```python
from build123d import *

# Parameters (mm, degrees)
ESBO_O1_W                = 180
ESBO_O1_H                = 80
RESSALTO_EXTRUS_O1_DEPTH = 2
ESBO_O2_R                = 1.5
CORTE_EXTRUS_O1_DEPTH    = 2
ESBO_O3_W                = 22
ESBO_O3_H                = 2.5
CORTE_EXTRUS_O2_DEPTH    = 2
FILETE4_R                = 1.25
FILETE5_R                = 1.25
FILETE6_R                = 1.25
FILETE7_R                = 1.25


with BuildPart() as part:
    # Esboço1 → Ressalto-extrusão1 (new body)
    with BuildSketch(Plane.XY):
        with Locations((90, -40)):
            Rectangle(ESBO_O1_W, ESBO_O1_H)
    extrude(amount=RESSALTO_EXTRUS_O1_DEPTH)

    # Esboço2 → Corte-extrusão1 (cut)
    with BuildSketch(Plane.XY.offset(2)):
        with Locations((5.5, -58.5)):
            Circle(ESBO_O2_R)
        with Locations((5.5, -21.5)):
            Circle(ESBO_O2_R)
        with Locations((174.5, -21.5)):
            Circle(ESBO_O2_R)
        with Locations((174.5, -58.5)):
            Circle(ESBO_O2_R)
    extrude(amount=-CORTE_EXTRUS_O1_DEPTH, mode=Mode.SUBTRACT)

    # Esboço3 → Corte-extrusão2 (cut)
    with BuildSketch(Plane.XY):
        with Locations((90, -12.25)):
            Rectangle(ESBO_O3_W, ESBO_O3_H)
        with Locations((90, -67.75)):
            Rectangle(ESBO_O3_W, ESBO_O3_H)
    extrude(amount=CORTE_EXTRUS_O2_DEPTH, mode=Mode.SUBTRACT)

    # Filete4
    filete4_edges = [part.edges().sort_by_distance(p)[0] for p in [
        (79, -11, 1),
        (79, -13.5, 1),
    ]]
    fillet(filete4_edges, radius=FILETE4_R - 0.0001)  # a hair under: the kernel refuses the full size

    # Filete5
    filete5_edges = [part.edges().sort_by_distance(p)[0] for p in [
        (101, -13.5, 1),
        (101, -11, 1),
    ]]
    fillet(filete5_edges, radius=FILETE5_R - 0.0001)  # a hair under: the kernel refuses the full size

    # Filete6
    filete6_edges = [part.edges().sort_by_distance(p)[0] for p in [
        (79, -66.5, 1),
        (79, -69, 1),
    ]]
    fillet(filete6_edges, radius=FILETE6_R - 0.0001)  # a hair under: the kernel refuses the full size

    # Filete7
    filete7_edges = [part.edges().sort_by_distance(p)[0] for p in [
        (101, -69, 1),
        (101, -66.5, 1),
    ]]
    fillet(filete7_edges, radius=FILETE7_R - 0.0001)  # a hair under: the kernel refuses the full size


solid = part.part
```
Model file for the job. Use its own axes, mm. Coordinates: 2 decimals unless noted, no trailing zeros. One line per item, written item: value. Start each with the question number.
1. Flat gauge pins, fed straight in: pin 1 (2.5 mm diameter, centred on x = 174.5, y = -21.5, fed in from -Z); pin 2 (5 mm diameter, centred on x = 81, y = -27, fed in from -Z). Where does each tip first touch, or does it go through?
2. Probe line 1 (Y direction, x = 5.5, z = 1.45); line 2 (Y direction, x = 100, z = 1); line 3 (X direction, y = -21, z = 1.3). List the from-to ranges inside material, lowest first. Write a range as from..to.
3. Mould opens along Y. For faces 1 (the flat face through (89, -39, 0)), 2 (the cylindrical face through (5.305, -20.013, 1.014)) say: released by +Y, released by -Y, zero draft, split by the parting line, or undercut.
Answers below:
1. pin 1: passes through
1. pin 2: stops at z = 0
2. line 1: y = -80..-60, -57..-23, -20..0
2. line 2: y = -80..-68.97, -66.53..-13.47, -11.03..0
2. line 3: x = 0..4.09, 6.91..173.09, 175.91..180
3. face 1: zero draft
3. face 2: undercut
